Build history of the part. All positions in model axes, mm. A direction names the side the tool comes from. Give positions to 0.01 mm unless a question says otherwise; leave off trailing zeros. Order: outer loops, then holes, each group sorted by start corner. A loop starts at its lowest first (then second) coordinate and runs counter-clockwise, first axis right, second up. Notation, with made-up numbers: (52, -32) -> (90, -32) arc R34 ccw to (90, 3) -> close; hole circle Ø11 at (89.5, 30.25). An arc over 180 degrees is marked (long way). Write item = value, one per line. Start each with the question number.
from build123d import *

# Parameters (mm, degrees)
F1_DEPTH = 8
F2_DEPTH = 1
F3_R     = 2.995
F3_R_2   = 2.495
F4_DEPTH = 1


with BuildPart() as f1:
    # F0 (on Front) → F1 (new body)
    with BuildSketch(Plane.XZ):
        with BuildLine():
            Line((3.4999999884, -7.8863207898), (3.4985407065, 10.0123348381))
            ThreePointArc((3.4985407065, 10.0123348381), (0.1392265828, 13.6106236093), (-3.495502424, 10.2907714275))
            Line((-3.495502424, 10.2907714275), (-3.4955897742, 9.9377461081))
            Line((-3.4955897742, 9.9377461081), (-3.4999998929, -7.8857401302))
            ThreePointArc((-3.4999998929, -7.8857401302), (-0.0002903298, -11.3866061336), (3.4999999884, -7.8863207898))
        make_face()
        with BuildLine():
            ThreePointArc((-2.9999999082, -7.8858638467), (0.0002488951, -4.8861127517), (2.99999999, -7.8863615549))
            ThreePointArc((2.99999999, -7.8863615549), (-0.0002488541, -10.8866061353), (-2.9999999082, -7.8858638467))
        make_face(mode=Mode.SUBTRACT)
        with BuildLine():
            ThreePointArc((2.9952903298, 1.1133938423), (2.1180751395, -1.0043909674), (0.0002903298, -1.8816061577))
            ThreePointArc((0.0002903298, -1.8816061577), (-2.1174944798, 3.231178652), (2.9952903298, 1.1133938423))
        make_face(mode=Mode.SUBTRACT)
        with BuildLine():
            ThreePointArc((2.9985313735, 10.0195343729), (0.0330453014, 7.0147601911), (-2.9958477024, 9.9556074667))
            ThreePointArc((-2.9958477024, 9.9556074667), (-0.031991606, 13.1132232724), (2.9985313735, 10.0195343729))
        make_face(mode=Mode.SUBTRACT)
        with BuildLine():
            ThreePointArc((2.9985313735, 10.0195343729), (-0.031991606, 13.1132232724), (-2.9958477024, 9.9556074667))
            ThreePointArc((-2.9958477024, 9.9556074667), (0.0330453014, 7.0147601911), (2.9985313735, 10.0195343729))
        make_face()
        with BuildLine():
            ThreePointArc((-2.4960813645, 9.9734690786), (-0.0266596741, 12.6132519269), (2.4984977744, 10.0267336432))
            ThreePointArc((2.4984977744, 10.0267336432), (0.0277133695, 7.5147315366), (-2.4960813645, 9.9734690786))
        make_face(mode=Mode.SUBTRACT)
        with BuildLine():
            ThreePointArc((2.9952903298, 1.1133938423), (-2.1174944798, 3.231178652), (0.0002903298, -1.8816061577))
            ThreePointArc((0.0002903298, -1.8816061577), (2.1180751395, -1.0043909674), (2.9952903298, 1.1133938423))
        make_face()
        with BuildLine():
            ThreePointArc((2.4952903298, 1.1133938423), (1.7645217489, -0.6508375768), (0.0002903298, -1.3816061577))
            ThreePointArc((0.0002903298, -1.3816061577), (-1.7639410893, 2.8776252614), (2.4952903298, 1.1133938423))
        make_face(mode=Mode.SUBTRACT)
        with BuildLine():
            ThreePointArc((-2.9999999082, -7.8858638467), (-0.0002488541, -10.8866061353), (2.99999999, -7.8863615549))
            ThreePointArc((2.99999999, -7.8863615549), (0.0002488951, -4.8861127517), (-2.9999999082, -7.8858638467))
        make_face()
        with BuildLine():
            ThreePointArc((-2.4999999235, -7.8859875632), (0.0002074125, -5.386194984), (2.4999999917, -7.88640232))
            ThreePointArc((2.4999999917, -7.88640232), (-0.0002073784, -10.3866061371), (-2.4999999235, -7.8859875632))
        make_face(mode=Mode.SUBTRACT)
    extrude(amount=F1_DEPTH)

    # F0 (on Front) → F2 (cut)
    with BuildSketch(Plane.XZ):
        with BuildLine():
            ThreePointArc((2.9985313735, 10.0195343729), (-0.031991606, 13.1132232724), (-2.9958477024, 9.9556074667))
            ThreePointArc((-2.9958477024, 9.9556074667), (0.0330453014, 7.0147601911), (2.9985313735, 10.0195343729))
        make_face()
        with BuildLine():
            ThreePointArc((-2.4960813645, 9.9734690786), (-0.0266596741, 12.6132519269), (2.4984977744, 10.0267336432))
            ThreePointArc((2.4984977744, 10.0267336432), (0.0277133695, 7.5147315366), (-2.4960813645, 9.9734690786))
        make_face(mode=Mode.SUBTRACT)
        with BuildLine():
            ThreePointArc((2.9952903298, 1.1133938423), (-2.1174944798, 3.231178652), (0.0002903298, -1.8816061577))
            ThreePointArc((0.0002903298, -1.8816061577), (2.1180751395, -1.0043909674), (2.9952903298, 1.1133938423))
        make_face()
        with BuildLine():
            ThreePointArc((2.4952903298, 1.1133938423), (1.7645217489, -0.6508375768), (0.0002903298, -1.3816061577))
            ThreePointArc((0.0002903298, -1.3816061577), (-1.7639410893, 2.8776252614), (2.4952903298, 1.1133938423))
        make_face(mode=Mode.SUBTRACT)
        with BuildLine():
            ThreePointArc((-2.9999999082, -7.8858638467), (-0.0002488541, -10.8866061353), (2.99999999, -7.8863615549))
            ThreePointArc((2.99999999, -7.8863615549), (0.0002488951, -4.8861127517), (-2.9999999082, -7.8858638467))
        make_face()
        with BuildLine():
            ThreePointArc((-2.4999999235, -7.8859875632), (0.0002074125, -5.386194984), (2.4999999917, -7.88640232))
            ThreePointArc((2.4999999917, -7.88640232), (-0.0002073784, -10.3866061371), (-2.4999999235, -7.8859875632))
        make_face(mode=Mode.SUBTRACT)
    extrude(amount=F2_DEPTH, mode=Mode.SUBTRACT)

    # F3 (on face) → F4 (cut)
    with BuildSketch(Plane.XZ.offset(8)):
        with BuildLine():
            ThreePointArc((2.9985313735, 10.0195343729), (-0.031991606, 13.1132232724), (-2.9958477024, 9.9556074667))
            ThreePointArc((-2.9958477024, 9.9556074667), (0.0330453014, 7.0147601911), (2.9985313735, 10.0195343729))
        make_face()
        with BuildLine():
            ThreePointArc((2.4984977744, 10.0267336432), (0.0277133695, 7.5147315366), (-2.4960813645, 9.9734690786))
            ThreePointArc((-2.4960813645, 9.9734690786), (-0.0266596741, 12.6132519269), (2.4984977744, 10.0267336432))
        make_face(mode=Mode.SUBTRACT)
        with Locations((0.0002903298, 1.1133938423)):
            Circle(F3_R)
        with Locations((0.0002903298, 1.1133938423)):
            Circle(F3_R_2, mode=Mode.SUBTRACT)
        with BuildLine():
            ThreePointArc((-2.9999999082, -7.8858638467), (-0.0002488541, -10.8866061353), (2.99999999, -7.8863615549))
            ThreePointArc((2.99999999, -7.8863615549), (0.0002488951, -4.8861127517), (-2.9999999082, -7.8858638467))
        make_face()
        with BuildLine():
            ThreePointArc((-2.4999999235, -7.8859875632), (0.0002074125, -5.386194984), (2.4999999917, -7.88640232))
            ThreePointArc((2.4999999917, -7.88640232), (-0.0002073784, -10.3866061371), (-2.4999999235, -7.8859875632))
        make_face(mode=Mode.SUBTRACT)
    extrude(amount=-F4_DEPTH, mode=Mode.SUBTRACT)


solid = f1.part
(1) Cut at C-C, the plane x = 1.5. Give the number of separate pieces and of enclosed holes in the cut face, plus the area to 3 significant figures.
(2) 3-axis set-ups, long thin cutter, end or side, ignore diameter. For faces 1 (the face through (0.036, -0.493, 13.113)), 2 (the face through (-2, 0, 4)), 3 (the face through (-2, -7, -6)), 4 (the face through (-0.083, -3.958, 12.612)): which of +Z, -Z, +X, -X, +Y, -Y reach the whole face in a straight line?
(3) Flat gauge pin, fed straight in: P1, Ø3, axis at y = -2, z = 2.5, coming from the -X side. Where does the tip first touch, or does it go through?
(4) Cut at A-A, the plane z = -8.5. Give the cut face in (x, y).
(5) Cut at B-B, the plane y = -5.5. Give the cut face in (x, z) (1 decimal), plus the area to 3 significant figures.
(6) Cut at D-D, the plane z = 11.75. Give the cut face in (x, y), plus the area to 3 significant figures.
(7) Wall check: line 1 (Z direction, x = 0, y = -3.75); line 2 (Z direction, x = -1.5, y = -2.75); line 3 (X direction, y = -3.5, z = 10). Give the ranges that are in metal, low to high. Write a range as [from, to].
(8) Mould opens along X. For faces 5 (the face through (0.216, -3.944, 13.607)), 6 (the face through (-2, -8, 4)), 7 (the face through (-2, -7, 3)), 8 (the face through (0.082, -3.958, 7.516)) say: released by +X, released by -X, zero draft, split by the parting line, or undercut.
Results:
q1.separate_pieces = 4
q1.enclosed_holes = 0
q1.area = 90.7 mm2
q2.face_1 = +Y
q2.face_2 = +Z, -Z, +X, -X, +Y
q2.face_3 = -Y
q2.face_4 = +Y, -Y
q3.P1 = -3.5
q4.outline = (-3.45, -8) -> (-2.94, -8) -> (-2.94, -7) -> (-2.42, -7) -> (-2.42, -1) -> (-2.94, -1) -> (-2.94, 0) -> (-3.45, 0) -> close; (2.42, -7) -> (2.94, -7) -> (2.94, -8) -> (3.45, -8) -> (3.45, 0) -> (2.94, 0) -> (2.94, -1) -> (2.42, -1) -> close
q5.outline = (-3.5, -7.9) arc R3.5 ccw to (3.5, -7.9) -> (3.5, 10) arc R3.5 ccw to (-3.5, 10.3) -> close; hole (-2.5, -7.9) arc R2.5 ccw to (2.5, -7.9) arc R2.5 ccw to start; hole circle Ø5 at (0, 1.1); hole (-2.5, 10) arc R2.5 ccw to (2.5, 10) arc R2.5 ccw (long way) to start
q5.area = 105 mm2
q6.outline = (-3.09, -8) -> (-2.51, -8) -> (-2.51, -7) -> (-1.89, -7) -> (-1.89, -1) -> (-2.51, -1) -> (-2.51, 0) -> (-3.09, 0) -> close; (1.89, -7) -> (2.51, -7) -> (2.51, -8) -> (3.09, -8) -> (3.09, 0) -> (2.51, 0) -> (2.51, -1) -> (1.89, -1) -> close
q6.area = 16.8 mm2
q7.line_1 = [-11.39, -10.39], [-5.39, -1.38], [3.61, 7.51], [12.61, 13.61]
q7.line_2 = [-11.05, -9.89], [-5.89, -0.88], [3.11, 8.02], [12.11, 13.28]
q7.line_3 = [-3.5, -2.5], [2.5, 3.5]
q8.face_5 = split by the parting line
q8.face_6 = zero draft
q8.face_7 = undercut
q8.face_8 = undercut
